from build123d import *

# Parameters (mm, degrees)
BOSS_EXTRUDE1_DEPTH = 10
BOSS_EXTRUDE2_DEPTH = 10


with BuildPart() as part:
    # Sketch2 → Boss-Extrude1 (new body)
    with BuildSketch(Plane.XY):
        with BuildLine():
            Line((0, 0), (250, 0))
            ThreePointArc((250, 0), (270, 20), (250, 40))
            Line((250, 40), (0, 40))
            Line((0, 40), (0, 0))
        make_face()
    extrude(amount=BOSS_EXTRUDE1_DEPTH)

    # Sketch3 → Boss-Extrude2 (add)
    with BuildSketch(Plane.XY.offset(10)):
        with BuildLine():
            ThreePointArc((250, 0), (260, 2.679491924), (267.320508076, 10))
            Line((267.320508076, 10), (115.043886481, 10))
            Line((115.043886481, 10), (0, 10))
            Line((0, 10), (0, 0))
            Line((0, 0), (250, 0))
        make_face()
        with BuildLine():
            ThreePointArc((269.364916731, 15), (270, 20), (269.364916731, 25))
            Line((269.364916731, 25), (0, 25))
            Line((0, 25), (0, 15))
            Line((0, 15), (269.364916731, 15))
        make_face()
        with BuildLine():
            ThreePointArc((267.320508076, 30), (260, 37.320508076), (250, 40))
            Line((250, 40), (0, 40))
            Line((0, 40), (0, 30))
            Line((0, 30), (267.320508076, 30))
        make_face()
    extrude(amount=BOSS_EXTRUDE2_DEPTH)


solid = part.part
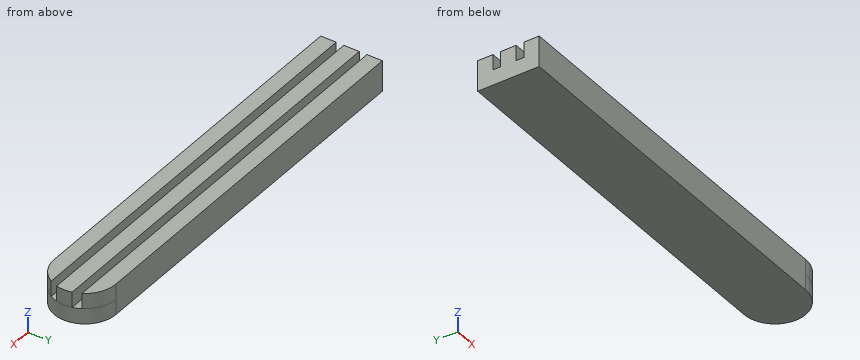
Check sheet for the modelled part. Datum: model origin and axes. Units: mm. Round coordinates to 2 decimals unless told otherwise and drop trailing zeros. Loops run counter-clockwise (first coordinate to the right, second up) from the corner with the lowest first, then second, coordinate; pieces in that order, holes last. Notation, with made-up numbers: (7, 25) -> (19, 25) arc R20 ccw to (19, 44) -> close; hole circle Ø6 at (-0.5, -38). An arc over 180 degrees is marked (long way). Put each result on its own line as item: value. Start each with the question number.
1. Scan lines: probe 1 along Y at (x, z) = (189, 13.75); probe 2 along Z at (x, y) = (231, 13); probe 3 along X at (y, z) = (16, 16.75). Record each from-to range of solid material in increasing order.
2. Section check A-A (z = 17.75). Enter the section's corners in (x, y), plus the area to 3 significant figures.
3. Section check C-C (y = 3). Enter the section's corners in (x, z), plus the area to 3 significant figures.
4. Section check B-B (x = 65). Enter the section's corners in (y, z), plus the area to 3 significant figures.
5. Gauge pin test, flat end, axial feed: pin 1 (10 mm diameter, centred on y = 5.5, z = 4, fed in from +X). Record the tip position at first contact, or that the pin passes through.
6. Section check D-D (z = 7.5). Enter the section's corners in (x, y).
Findings:
1. probe 1: y = 0 to 10, 15 to 25, 30 to 40
1. probe 2: z = 0 to 10
1. probe 3: x = 0 to 269.6
2. outline: (0, 0) -> (250, 0) arc R20 ccw to (267.32, 10) -> (0, 10) -> close; (0, 15) -> (269.36, 15) arc R20 ccw to (269.36, 25) -> (0, 25) -> close; (0, 30) -> (267.32, 30) arc R20 ccw to (250, 40) -> (0, 40) -> close
2. area: 7,940 mm^2
3. outline: (0, 0) -> (260.54, 0) -> (260.54, 20) -> (0, 20) -> close
3. area: 5,210 mm^2
4. outline: (0, 0) -> (40, 0) -> (40, 20) -> (30, 20) -> (30, 10) -> (25, 10) -> (25, 20) -> (15, 20) -> (15, 10) -> (10, 10) -> (10, 20) -> (0, 20) -> close
4. area: 700 mm^2
5. pin 1: stops at x = 267.6
6. outline: (0, 0) -> (250, 0) arc R20 ccw to (250, 40) -> (0, 40) -> close
